Here's how the part is built. I have some questions about the finished solid (model axes, mm). Round coordinates to 2 decimals unless told otherwise and drop trailing zeros. Write each loop counter-clockwise with the first axis right and the second up, starting at its lowest first coordinate (ties: lowest second). Pieces come first, ordered by that corner, then holes. Notation, with made-up numbers: (4.5, 13) -> (60.5, 13) arc R12 cw to (60.5, 24) -> close; hole circle Ø3 at (-30.5, 85). An arc over 180 degrees is marked (long way). Answer as CSV lines item,"result".
from build123d import *

# Parameters (mm, degrees)
F1_DEPTH = 508
F2_W     = 371.5004
F2_H     = 498.5004
F3_DEPTH = 25.4


with BuildPart() as f1:
    # F0 (on Front) → F1 (new body)
    with BuildSketch(Plane.XZ):
        Polygon((-175.6305839464, 61.4008368448), (-176.807737869, 53.0249514658), (200.4843963216, 0), (201.6615502441, 8.375885379), align=None)
    extrude(amount=-F1_DEPTH)

    # F2 (on face) → F3 (cut)
    with BuildSketch(Plane(origin=(5.0603666747, 0, 36.0063798214), x_dir=(0.9902680687, 0, -0.139173101), z_dir=(0.139173101, 0, 0.9902680687))):
        with Locations((8.0332959582, 254)):
            Rectangle(F2_W, F2_H)
    extrude(amount=-F3_DEPTH, mode=Mode.SUBTRACT)


solid = f1.part
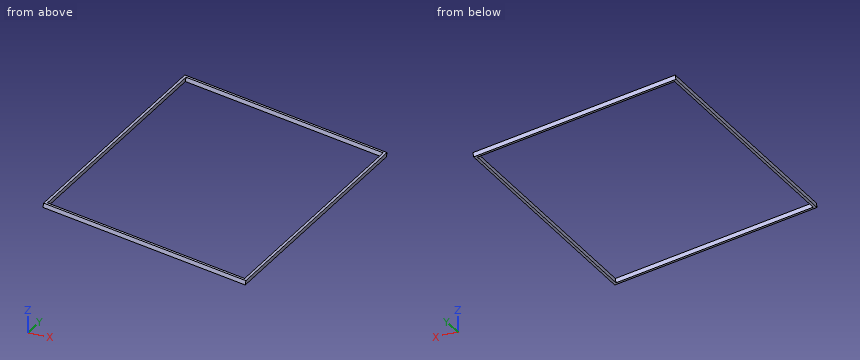
Item 1: Suppose I cut it at B-B, the plane z = 18.5. List the corners of the cut face in (x, y) for me, then the cut area to 3 significant figures.
Results found:
outline,"(68.85, 0) -> (129.62, 0) -> (129.62, 4.75) -> (68.85, 4.75) -> close; (68.85, 503.25) -> (129.62, 503.25) -> (129.62, 508) -> (68.85, 508) -> close"
area,"577 mm²"
Item 2: Suppose I cut it at A-A, the plane y = 419. List the corners of the cut face in (x, z) for me.
Results found:
outline,"(-176.81, 53.02) -> (-172.1, 52.36) -> (-170.93, 60.74) -> (-175.63, 61.4) -> close; (195.78, 0.66) -> (200.48, 0) -> (201.66, 8.38) -> (196.96, 9.04) -> close"
Item 3: I need wall thicknesses on L1, parallel to X at y = 323, z = 54; L2, parallel to X at y = 298, z = 55. Which ranges of each line are inside material? Lowest first, please.
Results found:
L1,"x = -176.67 to -171.87"
L2,"x = -176.53 to -171.73"
Item 4: Will this pin go through, and if not, where does the flat tip stop? pin 1 (10 mm diameter, centred on x = 105.5, z = 13, fed in from -Y).
Results found:
pin 1,"stops at y = 0"
